Here's how the part is built. I have some questions about the finished solid (model axes, mm). Round coordinates to 2 decimals unless told otherwise and drop trailing zeros. Write each loop counter-clockwise with the first axis right and the second up, starting at its lowest first coordinate (ties: lowest second). Pieces come first, ordered by that corner, then holes. Notation, with made-up numbers: (-26, -5.5) -> (20, -5.5) arc R20 cw to (20, 14.5) -> close; hole circle Ø11 at (33.25, 53). An arc over 180 degrees is marked (long way). Put each result on its own line as item: value. Start each with the question number.
1) If I drill on line 1 along X through (y, z) = (25, 2.2); line 2 along Y through (x, z) = (-0.8, 2.05); line 3 along Y through (x, z) = (0.55, 0.6), over which ranges is the centre line in solid material (lowest first)? Write a range as [from, to].
2) I want a section at A-A, the plane z = 3.75. List the corners of the cut face in (x, y) for me, then the cut area to 3 significant figures.
3) I want a section at B-B, the plane y = 45. List the corners of the cut face in (x, z) for me, then the cut area to 3 significant figures.
4) Will these pins go through, and if not, where does the flat tip stop? P1, Ø2, axis at x = -1.5, z = 1, coming from the +Y side; P2, Ø1.1, axis at x = -2, z = 1.5, coming from the +Y side.
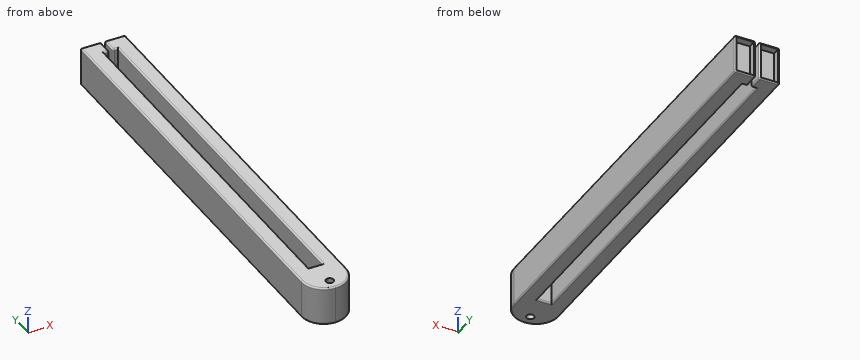
from build123d import *

# Parameters (mm, degrees)
F0_W     = 1.8
F0_H     = 50
F1_DEPTH = 5
F2_W     = 0.5
F2_H     = 5
F3_DEPTH = 2
F4_R     = 0.2
F5_DEPTH = 1


with BuildPart() as f1:
    # F0 (on Top) → F1 (new body)
    with BuildSketch(Plane.XY):
        Polygon((2, -2), (2, 52), (-3.8, 52), (-3.8, -2), (-0.9, -2), align=None)
        with Locations((-0.9, 25)):
            Rectangle(F0_W, F0_H, mode=Mode.SUBTRACT)
        with BuildLine():
            ThreePointArc((-0.9, -4.9), (1.1506096654, -4.0506096654), (2, -2))
            Line((2, -2), (-0.9, -2))
            Line((-0.9, -2), (-0.9, -2.95))
            ThreePointArc((-0.9, -2.95), (-0.5464466094, -3.0964466094), (-0.4, -3.45))
            ThreePointArc((-0.4, -3.45), (-0.5464466094, -3.8035533906), (-0.9, -3.95))
            Line((-0.9, -3.95), (-0.9, -4.9))
        make_face()
        with BuildLine():
            Line((-0.9, -2.95), (-0.9, -2))
            Line((-0.9, -2), (-3.8, -2))
            ThreePointArc((-3.8, -2), (-2.9506096654, -4.0506096654), (-0.9, -4.9))
            Line((-0.9, -4.9), (-0.9, -3.95))
            ThreePointArc((-0.9, -3.95), (-1.4, -3.45), (-0.9, -2.95))
        make_face()
    extrude(amount=F1_DEPTH)

    # F2 (on face) → F3 (cut)
    with BuildSketch(Plane(origin=(0, 52, 0), x_dir=(-1, 0, 0), z_dir=(0, 1, 0))):
        with Locations((0.9, 2.5)):
            Rectangle(F2_W, F2_H)
    extrude(amount=-F3_DEPTH, mode=Mode.SUBTRACT)

    # F4
    f4_edges = [f1.edges().sort_by_distance(p)[0] for p in [
        (2, 52, 2.5),
        (0.675, 52, 0),
        (0.675, 52, 5),
        (-2.475, 52, 5),
        (-3.8, 52, 2.5),
        (-2.475, 52, 0),
        (-0.65, 52, 2.5),
        (-1.15, 52, 2.5),
        (-1.15, 51, 5),
        (-0.65, 51, 5),
        (-0.65, 51, 0),
        (-1.15, 51, 0),
        (-1.475, 50, 0),
        (-1.15, 50, 2.5),
        (-0.325, 50, 0),
        (-0.65, 50, 2.5),
        (-1.475, 50, 5),
        (-0.325, 50, 5),
        (2, 25, 5),
        (2, 25, 0),
        (-1.8, 25, 5),
        (-1.8, 25, 0),
        (0, 25, 5),
        (0, 25, 0),
        (-0.9, 0, 0),
        (-0.9, 0, 5),
    ]]
    fillet(f4_edges, radius=F4_R)

    # F5 (cut): faces of the model
    f5_faces = [f1.faces().sort_by_distance(p)[0] for p in [
        (-2.475, 52, 2.5),
        (0.675, 52, 2.5),
    ]]
    extrude(f5_faces, amount=-F5_DEPTH, mode=Mode.SUBTRACT)


solid = f1.part
Findings:
1. line 1: x = [-3.8, -1.8], [0, 2]
1. line 2: y = [-4.9, -3.94], [-2.96, 0]
1. line 3: y = [-4.51, 51]
2. outline: (-3.8, -2) arc R2.9 ccw to (2, -2) -> (2, 51.8) arc R0.2 ccw to (1.8, 52) -> (1.8, 51) -> (-0.45, 51) -> (-0.45, 52) arc R0.2 ccw to (-0.65, 51.8) -> (-0.65, 50.2) arc R0.2 ccw to (-0.45, 50) -> (0, 50) -> (0, 0) -> (-1.8, 0) -> (-1.8, 50) -> (-1.35, 50) arc R0.2 ccw to (-1.15, 50.2) -> (-1.15, 51.8) arc R0.2 ccw to (-1.35, 52) -> (-1.35, 51) -> (-3.6, 51) -> (-3.6, 52) arc R0.2 ccw to (-3.8, 51.8) -> close; hole circle Ø1 at (-0.9, -3.45)
2. area: 230 mm2
3. outline: (-3.8, 0.2) arc R0.2 ccw to (-3.6, 0) -> (-2, 0) arc R0.2 ccw to (-1.8, 0.2) -> (-1.8, 4.8) arc R0.2 ccw to (-2, 5) -> (-3.6, 5) arc R0.2 ccw to (-3.8, 4.8) -> close; (0, 0.2) arc R0.2 ccw to (0.2, 0) -> (1.8, 0) arc R0.2 ccw to (2, 0.2) -> (2, 4.8) arc R0.2 ccw to (1.8, 5) -> (0.2, 5) arc R0.2 ccw to (0, 4.8) -> close
3. area: 19.9 mm2
4. P1: stops at y = 52
4. P2: stops at y = 51
